Part model, mm, in its own coordinate system. A direction names the side the tool comes from. Round coordinates to 2 decimals unless told otherwise and drop trailing zeros. Write each loop counter-clockwise with the first axis right and the second up, starting at its lowest first coordinate (ties: lowest second). Pieces come first, ordered by that corner, then holes. Notation, with made-up numbers: M 36,17 L 80,17 A20 cw 80,40 Z; hole C 43,-37.75 d9. An arc over 180 degrees is marked long. Answer as a JSON object with one key per item and string values. Group by question number.
1. Band-saw the part on A-A, the plane z = -1.5. Write the cut outline in (x, y), plus the area to 3 significant figures.
2. Band-saw the part on B-B, the plane z = -6.75. Count the separate pieces of the cut face and the enclosed holes in it, plus the area to 3 significant figures.
3. Two-plate mould, pull along X, no slides. Class faces 3 (the face through (-12.597, 0.277, -2.129)), 4 (the face through (29, 1.5, -3)), 5 (the face through (44, 0, -8)), 6 (the face through (2.3, -2.3, -3.4)): +X half, -X half, draft (parallel to the pull), parting line (faces both ways), or undercut.
4. Which spindle directions (+Z, -Z, +X, -X, +Y, -Y) get a long thin tool onto all of the face, cutting with end or side? Do faces 1 (the face through (24.38, -1.87, -2.56)), 2 (the face through (44, -12.6, -2)). Say none if no direction does.
5. Drill centre lines: line 1 (Y direction, x = 0, z = -1.1); line 2 (X direction, y = 0, z = -0.8); line 3 (Y direction, x = 46.5, z = -0.25). Where is each one in solid material? Low to high. Write a range as from..to.
6. Drop flat-ended pins along their axis: pin 1 (6.5 mm diameter, centred on x = 88.98, y = 0, fed in from -Z); pin 2 (1 mm diameter, centred on y = 2.5, z = -2.5, fed in from -X); pin 3 (1.5 mm diameter, centred on y = -8, z = -6, fed in from -X). Give the stop position or say it passes through.
from build123d import *

# Parameters (mm, degrees)
BOSS_EXTRUDE1_DEPTH  = 4.5
BOSS_EXTRUDE2_DEPTH  = 4
CHAMFER2_START       = -4.2
CHAMFER2_2_DEPTH     = 4.2
CHAMFER2_START_2     = -8
CHAMFER2_3_OUTLINE_R = 8.8
CHAMFER2_3_DEPTH     = 3.8
SKETCH7_R            = 3
CUT_EXTRUDE3_DEPTH   = 103.673405561
SKETCH8_R            = 5.25
CUT_EXTRUDE4_DEPTH   = 4.6
CUT_EXTRUDE5_DEPTH   = 5.2


with BuildPart() as part:
    # Sketch1 → Boss-Extrude1 (new body)
    with BuildSketch(Plane.XY):
        with BuildLine():
            Line((0, 12.6), (88.982814426, 12.6))
            ThreePointArc((88.982814426, 12.6), (101.582814426, 0), (88.982814426, -12.6))
            Line((88.982814426, -12.6), (0, -12.6))
            ThreePointArc((0, -12.6), (-12.6, 0), (0, 12.6))
        make_face()
    extrude(amount=-BOSS_EXTRUDE1_DEPTH)

    # Sketch2 → Boss-Extrude2 (add)
    with BuildSketch(Plane.XY.offset(-8)):
        with BuildLine():
            Line((89.741407213, 8.85), (-0.758592787, 8.85))
            ThreePointArc((-0.758592787, 8.85), (-9.608592787, 0), (-0.758592787, -8.85))
            Line((-0.758592787, -8.85), (89.741407213, -8.85))
            ThreePointArc((89.741407213, -8.85), (98.591407213, 0), (89.741407213, 8.85))
        make_face()
    extrude(amount=BOSS_EXTRUDE2_DEPTH)

    # Chamfer2: read off the stored shape, not the designer's step
    # Chamfer2 outline → Chamfer2 (revolve)
    with BuildSketch(Plane.XZ):
        Polygon((8.8, -4.2), (8.8, -8), (12.6, -4.2), align=None)
    revolve(axis=Axis((0, 0, 0), (0, 0, 1)))

    # Chamfer2 2 outline → Chamfer2 2 (add)
    with BuildSketch(Plane.XY.offset(CHAMFER2_START)):
        with BuildLine():
            Line((88.982814426, 12.6), (0, 12.6))
            ThreePointArc((0, 12.6), (-12.6, 0), (0, -12.6))
            Line((0, -12.6), (88.982814426, -12.6))
            ThreePointArc((88.982814426, -12.6), (101.582814426, 0), (88.982814426, 12.6))
        make_face()
    extrude(amount=CHAMFER2_2_DEPTH)

    # Chamfer2 3 outline → Chamfer2 3 (add)
    with BuildSketch(Plane.XY.offset(CHAMFER2_START_2)):
        Circle(CHAMFER2_3_OUTLINE_R)
    extrude(amount=CHAMFER2_3_DEPTH)

    # Chamfer2 4: loft between two sections, ruled curve by curve
    chamfer2_4_from = [
        Edge.make_three_point_arc((88.982814426, -8.8, -8), (95.205354101, -6.222539674, -8), (97.782814426, 0, -8)),
        Edge.make_three_point_arc((97.782814426, 0, -8), (95.205354101, 6.222539674, -8), (88.982814426, 8.8, -8)),
        Edge.make_line((0, 8.8, -8), (88.982814426, 8.8, -8)),
        Edge.make_line((88.982814426, -8.8, -8), (0, -8.8, -8)),
        Edge.make_line((0, -8.8, -8), (0, 8.8, -8)),
    ]
    chamfer2_4_to = [
        Edge.make_three_point_arc((88.982814426, -12.6, -4.2), (97.892359869, -8.909545443, -4.2), (101.582814426, 0, -4.2)),
        Edge.make_three_point_arc((101.582814426, 0, -4.2), (97.892359869, 8.909545443, -4.2), (88.982814426, 12.6, -4.2)),
        Edge.make_line((0, 12.6, -4.2), (88.982814426, 12.6, -4.2)),
        Edge.make_line((88.982814426, -12.6, -4.2), (0, -12.6, -4.2)),
        Edge.make_line((0, -12.6, -4.2), (0, 12.6, -4.2)),
    ]
    chamfer2_4 = Solid(Shell([*[Face.make_surface_from_curves(chamfer2_4_from[k], chamfer2_4_to[k]) for k in range(5)], Face(Wire(chamfer2_4_from)), Face(Wire(chamfer2_4_to))]))
    add(chamfer2_4)

    # Sketch7 → Cut-Extrude3 (cut, through all)
    with BuildSketch(Plane.XY.offset(-8)):
        Circle(SKETCH7_R)
        with Locations((88.982814426, 0)):
            Circle(SKETCH7_R)
    extrude(amount=CUT_EXTRUDE3_DEPTH, mode=Mode.SUBTRACT)

    # Sketch8 → Cut-Extrude4 (cut)
    with BuildSketch(Plane.XY.offset(-8)):
        Circle(SKETCH8_R)
        with Locations((88.982814426, 0)):
            Circle(SKETCH8_R)
    extrude(amount=CUT_EXTRUDE4_DEPTH, mode=Mode.SUBTRACT)

    # Sketch9 → Cut-Extrude5 (cut)
    with BuildSketch(Plane.XY):
        with BuildLine():
            Line((22.732649866, -2.964466094), (18.644187371, -7.052928589))
            Line((18.644187371, -7.052928589), (16.522867028, -4.931608246))
            Line((16.522867028, -4.931608246), (21.490009179, 0.035533906))
            ThreePointArc((21.490009179, 0.035533906), (23.112125923, 1.119397663), (25.025543085, 1.5))
            Line((25.025543085, 1.5), (33.8, 1.5))
            Line((33.8, 1.5), (33.8, 3.5))
            Line((33.8, 3.5), (36.6, 3.5))
            Line((36.6, 3.5), (36.6, 1.5))
            Line((36.6, 1.5), (43.021713367, 1.5))
            ThreePointArc((43.021713367, 1.5), (44.491407213, 2.1), (45.961101059, 1.5))
            Line((45.961101059, 1.5), (62.714630654, 1.5))
            ThreePointArc((62.714630654, 1.5), (64.628047816, 1.880602337), (66.25016456, 2.964466094))
            Line((66.25016456, 2.964466094), (70.338627055, 7.052928589))
            Line((70.338627055, 7.052928589), (72.459947399, 4.931608246))
            Line((72.459947399, 4.931608246), (67.492805247, -0.035533906))
            ThreePointArc((67.492805247, -0.035533906), (65.870688503, -1.119397663), (63.957271341, -1.5))
            Line((63.957271341, -1.5), (46.05578497, -1.5))
            Line((46.05578497, -1.5), (46.05578497, -2.91))
            Line((46.05578497, -2.91), (43.021713367, -2.91))
            Line((43.021713367, -2.91), (43.021713367, -1.5))
            Line((43.021713367, -1.5), (26.268183772, -1.5))
            ThreePointArc((26.268183772, -1.5), (24.35476661, -1.880602337), (22.732649866, -2.964466094))
        make_face()
    extrude(amount=-CUT_EXTRUDE5_DEPTH, mode=Mode.SUBTRACT)


solid = part.part
Worked answers:
{
 "1": {"outline": "M 0,-12.6 L 88.98,-12.6 A12.6 ccw 88.98,12.6 L 0,12.6 A12.6 ccw Z; hole C 0,0 d6; hole M 16.52,-4.93 L 18.64,-7.05 L 22.73,-2.96 A5 cw 26.27,-1.5 L 43.02,-1.5 L 43.02,-2.91 L 46.06,-2.91 L 46.06,-1.5 L 63.96,-1.5 A5 ccw 67.49,-0.04 L 72.46,4.93 L 70.34,7.05 L 66.25,2.96 A5 cw 62.71,1.5 L 45.96,1.5 A2.1 ccw 43.02,1.5 L 36.6,1.5 L 36.6,3.5 L 33.8,3.5 L 33.8,1.5 L 25.03,1.5 A5 ccw 21.49,0.04 Z; hole C 88.98,0 d6", "area": "2,500 mm^2"},
 "2": {"separate pieces": "1", "enclosed holes": "2", "area": "1,930 mm^2"},
 "3": {"face 3": "-X half", "face 4": "undercut", "face 5": "draft", "face 6": "undercut"},
 "4": {"face 1": "+Z", "face 2": "+Z, -Z, +X, -X, -Y"},
 "5": {"line 1": "y = -12.6..-3, 3..12.6", "line 2": "x = -12.6..-3, 3..21.45, 67.53..85.98, 91.98..101.58", "line 3": "y = -12.6..-1.5, 1.5..12.6"},
 "6": {"pin 1": "stops at z = -3.4", "pin 2": "stops at x = -12.44", "pin 3": "stops at x = -8.54"}
}
